CAD build for the part. Positions are in the model's coordinates, mm. Round coordinates to 2 decimals unless told otherwise and drop trailing zeros. Write each loop counter-clockwise with the first axis right and the second up, starting at its lowest first coordinate (ties: lowest second). Pieces come first, ordered by that corner, then holes. Notation, with made-up numbers: (40, -1.75) - (79, -1.75) arc R11 cw to (79, 12.25) - close; hole circle Ø10 at (66.5, 19.25). An arc over 180 degrees is marked (long way). Use one line per item in the form item = value. Start each with the question number.
Item 1: Drill centre lines: L1, parallel to X at y = 647, z = 3.85; L2, parallel to X at y = 614.5, z = 1.9; L3, parallel to Y at x = -633.5, z = 1.75. Where is each one in solid material? Low to high.
Item 2: Band-saw the part on A-A, the plane y = 642.5. List the corners of the cut face in (x, z).
Item 3: Band-saw the part on B-B, the plane z = 1.2. List the corners of the cut face in (x, y) (3 decimals).
Item 4: Band-saw the part on C-C, the plane y = 676.5. List the corners of the cut face in (x, z), and give its area (3 significant figures).
from build123d import *

# Parameters (mm, degrees)
SKETCH1_R           = 2.921
SKETCH1_R_2         = 3.175
BOSS_EXTRUDE1_DEPTH = 5.9944


with BuildPart() as part:
    # Sketch1 → Boss-Extrude1 (new body)
    with BuildSketch(Plane(origin=(0, 0, 0), x_dir=(-1, 0, 0), z_dir=(0, 0, 1))):
        with BuildLine():
            Line((566.61706408, -610.968899583), (566.61706408, -679.368899583))
            ThreePointArc((566.61706408, -679.368899583), (568.081530174, -682.904433489), (571.61706408, -684.368899583))
            Line((571.61706408, -684.368899583), (637.01706408, -684.368899583))
            ThreePointArc((637.01706408, -684.368899583), (640.552597986, -682.904433489), (642.01706408, -679.368899583))
            Line((642.01706408, -679.368899583), (642.01706408, -610.968899583))
            ThreePointArc((642.01706408, -610.968899583), (640.552597986, -607.433365677), (637.01706408, -605.968899583))
            Line((637.01706408, -605.968899583), (571.61706408, -605.968899583))
            ThreePointArc((571.61706408, -605.968899583), (568.081530174, -607.433365677), (566.61706408, -610.968899583))
        make_face()
        with Locations((572.96706408, -612.318899583)):
            Circle(SKETCH1_R, mode=Mode.SUBTRACT)
        with Locations((635.66706408, -612.318899583)):
            Circle(SKETCH1_R_2, mode=Mode.SUBTRACT)
        with Locations((635.66706408, -678.018899583)):
            Circle(SKETCH1_R_2, mode=Mode.SUBTRACT)
        with Locations((572.96706408, -678.018899583)):
            Circle(SKETCH1_R_2, mode=Mode.SUBTRACT)
        with BuildLine():
            ThreePointArc((587.220270562, -660.668899583), (589.31706408, -662.765693101), (591.413857599, -660.668899583))
            Line((591.413857599, -660.668899583), (591.413857599, -630.668899583))
            ThreePointArc((591.413857599, -630.668899583), (589.31706408, -628.572106065), (587.220270562, -630.668899583))
            Line((587.220270562, -630.668899583), (587.220270562, -660.668899583))
        make_face(mode=Mode.SUBTRACT)
        with BuildLine():
            ThreePointArc((617.214915153, -660.668899583), (619.31706408, -662.771048511), (621.419213008, -660.668899583))
            Line((621.419213008, -660.668899583), (621.419213008, -630.668899583))
            ThreePointArc((621.419213008, -630.668899583), (619.31706408, -628.566750655), (617.214915153, -630.668899583))
            Line((617.214915153, -630.668899583), (617.214915153, -660.668899583))
        make_face(mode=Mode.SUBTRACT)
    extrude(amount=BOSS_EXTRUDE1_DEPTH)


solid = part.part
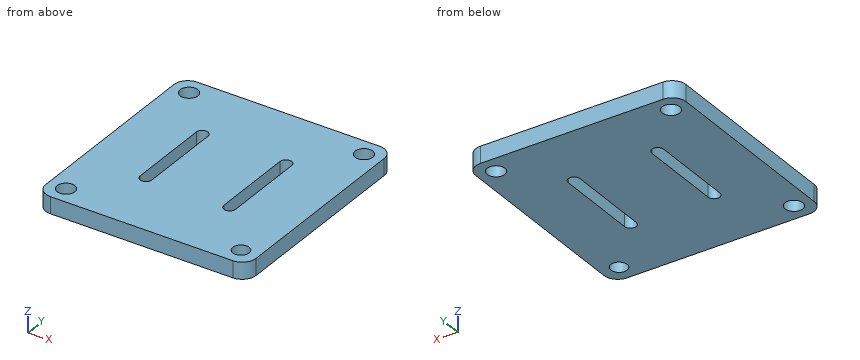
Determined:
q1.L1 = -642.02 to -621.42, -617.21 to -591.41, -587.22 to -566.62
q1.L2 = -642.02 to -637.97, -633.36 to -574.91, -571.02 to -566.62
q1.L3 = 605.97 to 610, 614.64 to 675.7, 680.34 to 684.37
q2.outline = (-642.02, 0) - (-621.42, 0) - (-621.42, 5.99) - (-642.02, 5.99) - close; (-617.21, 0) - (-591.41, 0) - (-591.41, 5.99) - (-617.21, 5.99) - close; (-587.22, 0) - (-566.62, 0) - (-566.62, 5.99) - (-587.22, 5.99) - close
q3.outline = (-642.017, 610.969) arc R5 ccw to (-637.017, 605.969) - (-571.617, 605.969) arc R5 ccw to (-566.617, 610.969) - (-566.617, 679.369) arc R5 ccw to (-571.617, 684.369) - (-637.017, 684.369) arc R5 ccw to (-642.017, 679.369) - close; hole circle Ø6.35 at (-635.667, 612.319); hole circle Ø6.35 at (-635.667, 678.019); hole (-621.419, 630.669) arc R2.102 ccw to (-617.215, 630.669) - (-617.215, 660.669) arc R2.102 ccw to (-621.419, 660.669) - close; hole (-591.414, 630.669) arc R2.097 ccw to (-587.22, 630.669) - (-587.22, 660.669) arc R2.097 ccw to (-591.414, 660.669) - close; hole circle Ø6.35 at (-572.967, 678.019); hole circle Ø5.842 at (-572.967, 612.319)
q4.outline = (-642.02, 0) - (-638.46, 0) - (-638.46, 5.99) - (-642.02, 5.99) - close; (-632.88, 0) - (-575.76, 0) - (-575.76, 5.99) - (-632.88, 5.99) - close; (-570.18, 0) - (-566.62, 0) - (-566.62, 5.99) - (-570.18, 5.99) - close
q4.area = 385 mm²
